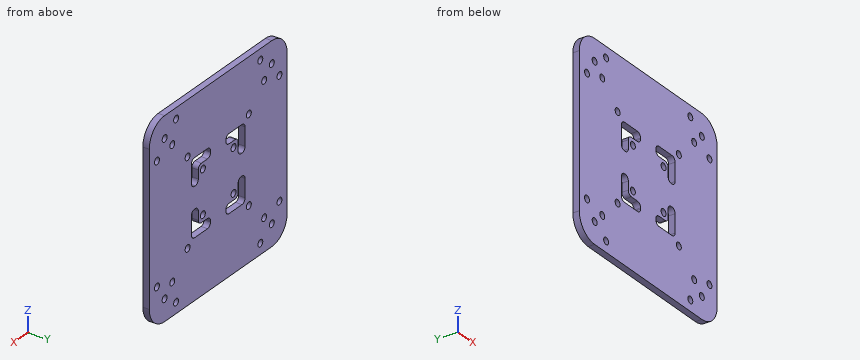
from build123d import *

# Parameters (mm, degrees)
SKETCH_1_W          = 90
SKETCH_1_H          = 90
SKETCH_1_R          = 1.6
EXTRUDE_1_DEPTH     = 3
SKETCH_3_R          = 1.6
CUT_EXTRUDE_2_DEPTH = 64.710281745
FILLET_1_R          = 2
FILLET_3_R          = 10
SKETCH_6_R          = 1.6
CUT_EXTRUDE_4_DEPTH = 64.710281745
SKETCH_12_R         = 1.6
CUT_EXTRUDE_5_DEPTH = 64.710281745


with BuildPart() as part:
    # 草图1 → 凸台-拉伸1 (new body)
    with BuildSketch(Plane(origin=(0, 0, 0), x_dir=(1, 0, 0), z_dir=(0, 1, 0))):
        Rectangle(SKETCH_1_W, SKETCH_1_H)
        with Locations(Location((-35, -35, 0), (0, 0, 270))):
            Circle(SKETCH_1_R, mode=Mode.SUBTRACT)
        with Locations(Location((35, -35, 0), (0, 0, 270))):
            Circle(SKETCH_1_R, mode=Mode.SUBTRACT)
        Polygon((17.5, -17.5), (5, -17.5), (5, -13), (13, -13), (13, -5), (17.5, -5), align=None, mode=Mode.SUBTRACT)
        Polygon((-13, -13), (-5, -13), (-5, -17.5), (-17.5, -17.5), (-17.5, -5), (-13, -5), align=None, mode=Mode.SUBTRACT)
        Polygon((-17.5, 5), (-17.5, 17.5), (-5, 17.5), (-5, 13), (-13, 13), (-13, 5), align=None, mode=Mode.SUBTRACT)
        Polygon((5, 17.5), (17.5, 17.5), (17.5, 5), (13, 5), (13, 13), (5, 13), align=None, mode=Mode.SUBTRACT)
        with Locations(Location((-35, 35, 0), (0, 0, 270))):
            Circle(SKETCH_1_R, mode=Mode.SUBTRACT)
        with Locations(Location((35, 35, 0), (0, 0, 270))):
            Circle(SKETCH_1_R, mode=Mode.SUBTRACT)
        with Locations(Location((10, -10, 0), (0, 0, 270))):
            Circle(SKETCH_1_R, mode=Mode.SUBTRACT)
        with Locations(Location((-10, -10, 0), (0, 0, 270))):
            Circle(SKETCH_1_R, mode=Mode.SUBTRACT)
        with Locations(Location((10, 10, 0), (0, 0, 270))):
            Circle(SKETCH_1_R, mode=Mode.SUBTRACT)
        with Locations(Location((-10, 10, 0), (0, 0, 270))):
            Circle(SKETCH_1_R, mode=Mode.SUBTRACT)
    extrude(amount=EXTRUDE_1_DEPTH)

    # 草图3 → 切除-拉伸2 (cut, through all)
    with BuildSketch(Plane(origin=(0, 3, 0), x_dir=(1, 0, 0), z_dir=(0, 1, 0))):
        with Locations(Location((-20, 20, 0), (0, 0, 270))):
            Circle(SKETCH_3_R)
        with Locations(Location((20, 20, 0), (0, 0, 270))):
            Circle(SKETCH_3_R)
        with Locations(Location((20, -20, 0), (0, 0, 270))):
            Circle(SKETCH_3_R)
        with Locations(Location((-20, -20, 0), (0, 0, 270))):
            Circle(SKETCH_3_R)
    extrude(amount=-CUT_EXTRUDE_2_DEPTH, mode=Mode.SUBTRACT)

    # 圆角1
    fillet_1_edges = [part.edges().sort_by_distance(p)[0] for p in [
        (17.5, 1.5, 17.5),
        (17.5, 1.5, 5),
        (13, 1.5, 5),
        (13, 1.5, 13),
        (5, 1.5, 13),
        (5, 1.5, 17.5),
        (-5, 1.5, 13),
        (-13, 1.5, 13),
        (-13, 1.5, 5),
        (-17.5, 1.5, 5),
        (-17.5, 1.5, 17.5),
        (-5, 1.5, 17.5),
        (-5, 1.5, -17.5),
        (-17.5, 1.5, -17.5),
        (-17.5, 1.5, -5),
        (-13, 1.5, -5),
        (-13, 1.5, -13),
        (-5, 1.5, -13),
        (17.5, 1.5, -5),
        (17.5, 1.5, -17.5),
        (5, 1.5, -17.5),
        (5, 1.5, -13),
        (13, 1.5, -13),
        (13, 1.5, -5),
    ]]
    fillet(fillet_1_edges, radius=FILLET_1_R)

    # 圆角3
    fillet_3_edges = [part.edges().sort_by_distance(p)[0] for p in [
        (-45, 1.5, -45),
        (45, 1.5, -45),
        (45, 1.5, 45),
        (-45, 1.5, 45),
    ]]
    fillet(fillet_3_edges, radius=FILLET_3_R)

    # 草图6 → 切除-拉伸4 (cut, through all)
    with BuildSketch(Plane(origin=(0, 3, 0), x_dir=(1, 0, 0), z_dir=(0, 1, 0))):
        with Locations(Location((-27.5, 40, 0), (0, 0, 270))):
            Circle(SKETCH_6_R)
        with Locations(Location((27.5, 40, 0), (0, 0, 270))):
            Circle(SKETCH_6_R)
        with Locations(Location((40, 27.5, 0), (0, 0, 270))):
            Circle(SKETCH_6_R)
        with Locations(Location((27.5, -40, 0), (0, 0, 270))):
            Circle(SKETCH_6_R)
        with Locations(Location((-40, -27.5, 0), (0, 0, 270))):
            Circle(SKETCH_6_R)
        with Locations(Location((40, -27.5, 0), (0, 0, 270))):
            Circle(SKETCH_6_R)
        with Locations(Location((-27.5, -40, 0), (0, 0, 270))):
            Circle(SKETCH_6_R)
        with Locations(Location((-40, 27.5, 0), (0, 0, 270))):
            Circle(SKETCH_6_R)
    extrude(amount=-CUT_EXTRUDE_4_DEPTH, mode=Mode.SUBTRACT)

    # 草图12 → 切除-拉伸5 (cut, through all)
    with BuildSketch(Plane(origin=(0, 3, 0), x_dir=(1, 0, 0), z_dir=(0, 1, 0))):
        with Locations(Location((-30, 30, 0), (0, 0, 270))):
            Circle(SKETCH_12_R)
        with Locations(Location((30, 30, 0), (0, 0, 270))):
            Circle(SKETCH_12_R)
        with Locations(Location((30, -30, 0), (0, 0, 270))):
            Circle(SKETCH_12_R)
        with Locations(Location((-30, -30, 0), (0, 0, 270))):
            Circle(SKETCH_12_R)
    extrude(amount=-CUT_EXTRUDE_5_DEPTH, mode=Mode.SUBTRACT)


solid = part.part
Check sheet for the modelled part. Datum: model origin and axes. Units: mm. Give positions to 0.01 mm unless a question says otherwise; leave off trailing zeros. Order: outer loops, then holes, each group sorted by start corner. A loop starts at its lowest first (then second) coordinate and runs counter-clockwise, first axis right, second up. Notation, with made-up numbers: (32, -15.75) - (42, -15.75) arc R12 cw to (42, -7.75) - close; hole circle Ø6 at (29, 62.5). An arc over 180 degrees is marked (long way). Answer as CSV lines item,"result".
1. Section check C-C (y = 0.9). State how many separate pieces and enclosed holes the cut face has, then the cut area to 3 significant figures.
Result sheet:
separate pieces,"1"
enclosed holes,"28"
area,"7,470 mm²"
2. Section check A-A (z = 20). Record the boundary of the cut face in (x, y).
Result sheet:
outline,"(-45, 0) - (-21.6, 0) - (-21.6, 3) - (-45, 3) - close; (-18.4, 0) - (18.4, 0) - (18.4, 3) - (-18.4, 3) - close; (21.6, 0) - (45, 0) - (45, 3) - (21.6, 3) - close"
3. Scan lines: probe 1 along X at (y, z) = (1.55, 20); probe 2 along Z at (x, y) = (-8, 0.4); probe 3 along X at (y, z) = (0.75, -10). Record each from-to range of solid material in increasing order. Write a range as from..to.
Result sheet:
probe 1,"-45..-21.6, -18.4..18.4, 21.6..45"
probe 2,"-45..-17.5, -13..13, 17.5..45"
probe 3,"-45..-17.5, -13..-11.6, -8.4..8.4, 11.6..13, 17.5..45"
4. Section check B-B (x = -20). Record the boundary of the cut face in (y, z).
Result sheet:
outline,"(0, -45) - (3, -45) - (3, -21.6) - (0, -21.6) - close; (0, -18.4) - (3, -18.4) - (3, 18.4) - (0, 18.4) - close; (0, 21.6) - (3, 21.6) - (3, 45) - (0, 45) - close"
